Could you check a few things on this model? Use its own coordinates, in mm. A direction names the side the tool comes from. Round coordinates to 2 decimals unless told otherwise and drop trailing zeros. Write each loop counter-clockwise with the first axis right and the second up, starting at its lowest first coordinate (ties: lowest second). Pieces come first, ordered by that corner, then holes. Notation, with made-up numbers: M 31,-22 L 82,-22 A15 ccw 82,-9 Z; hole C 34.5,-17 d2. An arc over 180 degrees is marked long. One line per item, written item: value. Start each with the question number.
(1) I want a section at D-D on x = -1. Please give me the cut outline in (y, z), and give its area (3 significant figures).
(2) Which directions (+Z, -Z, +X, -X, +Y, -Y) give clear straight access to the entire face, cutting with the end or side of a thin tool? Please do faces 4 (the face through (-11.232, 0.872, 15.526)), 5 (the face through (11.23, -7.26, 7.42)), 6 (the face through (0, 0, 0)).
(3) Thinking about a two-plate mould opening in Y: for faces 1 (the face through (-12.5, 0, 6)), 2 (the face through (-11.232, -0.896, 15.501)), 3 (the face through (0, 10, -1)), which applies, released by +Y, released by -Y, zero draft, split by the parting line, or undercut?
(4) I want a section at C-C on z = 15. Please give me the cut outline in (x, y), and give its area (3 significant figures).
(5) I want a section at B-B on y = -2.5. Please give me the cut outline in (x, z).
(6) I want a section at A-A on z = 1.5. Please give me the cut outline in (x, y), and give its area (3 significant figures).
(7) If I drill on L1, parallel to X at y = 6, z = 10.5; L2, parallel to Z at x = 1.5, y = -7.25; L3, parallel to Y at x = -11.5, z = 16, over which ranges is the centre line in solid material (lowest first)?
(8) I'm going to push a flat-ended pin straight in: pin 1 Ø10 at (x, y) = (1.5, -1.5) entering from +Z. Where does the tip first touch, or does it pass through?
```python
from build123d import *

# Parameters (mm, degrees)
F2_DEPTH = 2.5
F3_W     = 25
F3_H     = 20
F4_DEPTH = 2


# Not quite as in the source:
# - a pattern or mirror of a feature is missing from the dataset's text; its kind, count and spacing are read off the source's solid


with BuildPart() as f2:
    # F1 (on offset) → F2 (new body)
    with BuildSketch(Plane.YZ.offset(10)):
        Polygon((-4.5961940777, 14.6293006837), (-10, 0), (10, 0), (4.5961940777, 14.6293006837), (0, 19.2254947614), align=None)
        Polygon((0, 16.3970676367), (1.767766953, 14.6293006837), (0, 12.8615337308), (-1.767766953, 14.6293006837), align=None, mode=Mode.SUBTRACT)
    extrude(amount=F2_DEPTH)


with BuildPart() as f2_copies_1:
    # F2_copies: instance of F2
    add(f2.part.mirror(Plane(origin=(0, 0, 0), x_dir=(0, 0, -1), z_dir=(-1, 0, 0))))


with BuildPart() as f2_1:
    add(f2.part)

    add(f2_copies_1.part)  # F4 merges F2_copies_1
    # F3 (on Top) → F4 (join)
    with BuildSketch(Plane.XY):
        Rectangle(F3_W, F3_H)
    extrude(amount=-F4_DEPTH)


solid = f2_1.part
```
Found:
1. outline: M -10,-2 L 10,-2 L 10,0 L -10,0 Z
1. area: 40.0 mm²
2. face 4: +X, -X
2. face 5: +Z, +X, -X, -Y
2. face 6: +Z, +Y, -Y
3. face 1: zero draft
3. face 2: undercut
3. face 3: released by +Y
4. outline: M -12.5,-4.23 L -10,-4.23 L -10,-1.4 L -12.5,-1.4 Z; M -12.5,1.4 L -10,1.4 L -10,4.23 L -12.5,4.23 Z; M 10,-4.23 L 12.5,-4.23 L 12.5,-1.4 L 10,-1.4 Z; M 10,1.4 L 12.5,1.4 L 12.5,4.23 L 10,4.23 Z
4. area: 28.3 mm²
5. outline: M -12.5,-2 L 12.5,-2 L 12.5,16.73 L 10,16.73 L 10,0 L -10,0 L -10,16.73 L -12.5,16.73 Z
6. outline: M -12.5,-9.45 L -10,-9.45 L -10,9.45 L -12.5,9.45 Z; M 10,-9.45 L 12.5,-9.45 L 12.5,9.45 L 10,9.45 Z
6. area: 94.5 mm²
7. L1: x = -12.5 to -10, 10 to 12.5
7. L2: z = -2 to 0
7. L3: y = -3.23 to -0.4, 0.4 to 3.23
8. pin 1: stops at z = 0
